Here's how the part is built. I have some questions about the finished solid (model axes, mm). Face numbers are marked on the shaded views. A direction names the side the tool comes from. Round coordinates to 2 decimals unless told otherwise and drop trailing zeros. Write each loop counter-clockwise with the first axis right and the second up, starting at its lowest first coordinate (ties: lowest second). Pieces come first, ordered by that corner, then holes. Notation, with made-up numbers: M 18.25,-6 L 23.25,-6 A31 cw 23.25,20 Z; hole C -15.5,51 d4. An arc over 180 degrees is marked long. Write item = value, one per line. Start each with the question number.
(1) I need wall thicknesses on line 1 along Y through (x, z) = (0, 10.5); line 2 along Z through (x, y) = (4.75, -1.25); line 3 along X through (y, z) = (-1.25, 9.5). Which ranges of each line are inside material? Lowest first, please.
(2) On a 3-axis mill with a long thin cutter (end or side, diameter ignored), from which of +Z, -Z, +X, -X, +Y, -Y can I reach the whole of each face in a straight line? I mean the marked faces 1 and 2. Say none if no direction works.
(3) Will these pins go through, and if not, where does the flat tip stop? pin 1 Ø1 at (x, z) = (-3.5, 5.5) entering from -Y; pin 2 Ø4 at (y, z) = (-3.5, 9.5) entering from +X; pin 3 Ø2 at (x, y) = (-3, -5.5) entering from +Z.
(4) I want a section at D-D (y = 3). List the corners of the cut face in (x, z) for me.
(5) I want a section at A-A (y = 0). List the corners of the cut face in (x, z) for me, and give its area (3 significant figures).
(6) I want a section at C-C (z = 6.5). List the corners of the cut face in (x, y) for me, and give its area (3 significant figures).
```python
from build123d import *

# Parameters (mm, degrees)
ESBO_O1_R                  = 12.15
RESSALTO_EXTRUS_O1_DEPTH   = 15
ESBO_O2_R                  = 4.5
RESSALTO_EXTRUS_O2_DEPTH   = 15.5
ESBO_O3_R                  = 1.554984666
CORTE_EXTRUS_O1_DEPTH      = 19.5
CORTE_EXTRUS_O1_DEPTH_BACK = 15.5


with BuildPart() as part:
    # Esboço1 → Ressalto-extrusão1 (new body)
    with BuildSketch(Plane.XY):
        Circle(ESBO_O1_R)
    extrude(amount=RESSALTO_EXTRUS_O1_DEPTH)

    # Esboço2 → Ressalto-extrusão2 (add)
    with BuildSketch(Plane.XY):
        Circle(ESBO_O2_R)
    extrude(amount=RESSALTO_EXTRUS_O2_DEPTH)

    # Esboço3 → Corte-extrusão1 (cut, two sides)
    with BuildSketch(Plane.XY) as corte_extrus_o1_sk:
        Circle(ESBO_O3_R)
    extrude(amount=CORTE_EXTRUS_O1_DEPTH, mode=Mode.SUBTRACT)
    extrude(corte_extrus_o1_sk.sketch, amount=-CORTE_EXTRUS_O1_DEPTH_BACK, mode=Mode.SUBTRACT)


solid = part.part
```
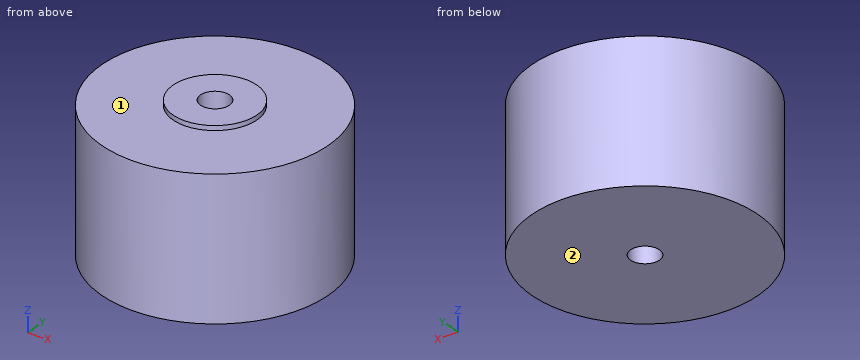
Returned:
q1.line_1 = -12.15 to -1.55, 1.55 to 12.15
q1.line_2 = 0 to 15
q1.line_3 = -12.09 to -0.92, 0.92 to 12.09
q2.face_1 = +Z
q2.face_2 = -Z, +X, -X, +Y, -Y
q3.pin_1 = -11.77
q3.pin_2 = 12.06
q3.pin_3 = 15
q4.outline = M -11.77,0 L 11.77,0 L 11.77,15 L 3.35,15 L 3.35,15.5 L -3.35,15.5 L -3.35,15 L -11.77,15 Z
q5.outline = M -12.15,0 L -1.55,0 L -1.55,15.5 L -4.5,15.5 L -4.5,15 L -12.15,15 Z; M 1.55,0 L 12.15,0 L 12.15,15 L 4.5,15 L 4.5,15.5 L 1.55,15.5 Z
q5.area = 321 mm²
q6.outline = C 0,0 d24.3; hole C 0,0 d3.11
q6.area = 456 mm²
